```python
from build123d import *

# Parameters (mm, degrees)
SKETCH1_R           = 1.75
BOSS_EXTRUDE1_DEPTH = 6.25


with BuildPart() as part:
    # Sketch1 → Boss-Extrude1 (new, symmetric)
    with BuildSketch(Plane(origin=(0, 0, 0), x_dir=(1, 0, 0), z_dir=(0, 1, 0))):
        with Locations(Location((0, 0, 0), (0, 0, 270))):
            Circle(SKETCH1_R)
    extrude(amount=BOSS_EXTRUDE1_DEPTH, both=True)

    # Sketch2 → Revolve1 (revolve)
    with BuildSketch(Plane.XY, mode=Mode.PRIVATE) as revolve1_sk:
        with BuildLine():
            Line((-2.8, 6.25), (0, 6.25))
            Line((0, 6.25), (0, 7.75))
            Line((0, 7.75), (-2.8, 7.75))
            ThreePointArc((-2.8, 7.75), (-2.941421356, 7.691421356), (-3, 7.55))
            Line((-3, 7.55), (-3, 6.45))
            ThreePointArc((-3, 6.45), (-2.941421356, 6.308578644), (-2.8, 6.25))
        make_face()
        with BuildLine():
            Line((-2.8, -7.75), (0, -7.75))
            Line((0, -7.75), (0, -6.25))
            Line((0, -6.25), (-2.8, -6.25))
            ThreePointArc((-2.8, -6.25), (-2.941421356, -6.308578644), (-3, -6.45))
            Line((-3, -6.45), (-3, -7.55))
            ThreePointArc((-3, -7.55), (-2.941421356, -7.691421356), (-2.8, -7.75))
        make_face()
    revolve(revolve1_sk.sketch.rotate(Axis((0, -7.75, 0), (0, 1, 0)), 270), axis=Axis((0, -7.75, 0), (0, 1, 0)))


solid = part.part
```
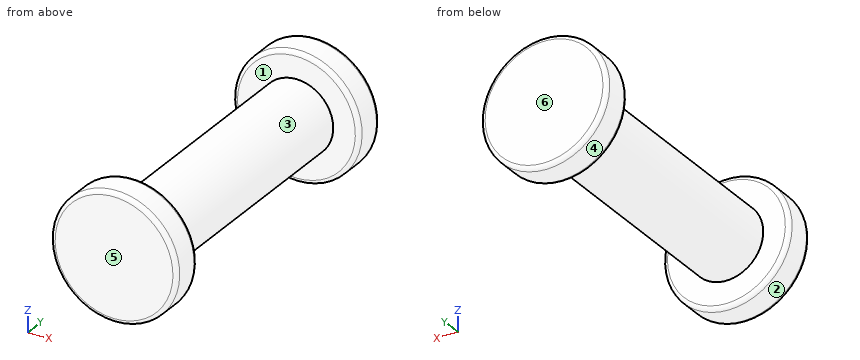
Here's how the part is built. I have some questions about the finished solid (model axes, mm). Face numbers are marked on the shaded views. A direction names the side the tool comes from. Round coordinates to 2 decimals unless told otherwise and drop trailing zeros. Loops run counter-clockwise (first coordinate to the right, second up) from the corner with the lowest first, then second, coordinate; pieces in that order, holes last.
1. Suppose I cut it at C-C, the plane y = -0.5. Please give me the cut outline in (x, z).
Answers:
outline: circle Ø3.5 at (0, 0)
2. Thinking about a two-plate mould opening in Y: for the marked faces 3, 4, 5 and 6, which applies, released by +Y, released by -Y, zero draft, split by the parting line, or undercut?
Answers:
face 3: undercut
face 4: zero draft
face 5: released by -Y
face 6: released by +Y
3. Suppose I cut it at A-A, the plane x = 0. Please give me the cut outline in (y, z).
Answers:
outline: (-7.75, -2.8) arc R0.2 ccw to (-7.55, -3) - (-6.45, -3) arc R0.2 ccw to (-6.25, -2.8) - (-6.25, -1.75) - (6.25, -1.75) - (6.25, -2.8) arc R0.2 ccw to (6.45, -3) - (7.55, -3) arc R0.2 ccw to (7.75, -2.8) - (7.75, 2.8) arc R0.2 ccw to (7.55, 3) - (6.45, 3) arc R0.2 ccw to (6.25, 2.8) - (6.25, 1.75) - (-6.25, 1.75) - (-6.25, 2.8) arc R0.2 ccw to (-6.45, 3) - (-7.55, 3) arc R0.2 ccw to (-7.75, 2.8) - close
4. For the marked faces 1 and 2, which set-ups out of +Z, -Z, +X, -X, +Y, -Y let a thin tool reach every point of the face, with its end or its side?
Answers:
face 1: none
face 2: +Y, -Y
5. If I drill on probe 1 along Y at (x, z) = (1.5, -1.5); probe 2 along X at (y, z) = (-5, 0.25); probe 3 along X at (y, z) = (-4.5, -1), over which ranges is the centre line in solid material (lowest first)?
Answers:
probe 1: y = -7.75 to -6.25, 6.25 to 7.75
probe 2: x = -1.73 to 1.73
probe 3: x = -1.44 to 1.44
6. Suppose I cut it at B-B, the plane z = 0. Please give me the cut outline in (x, y).
Answers:
outline: (-3, -7.55) arc R0.2 ccw to (-2.8, -7.75) - (2.8, -7.75) arc R0.2 ccw to (3, -7.55) - (3, -6.45) arc R0.2 ccw to (2.8, -6.25) - (1.75, -6.25) - (1.75, 6.25) - (2.8, 6.25) arc R0.2 ccw to (3, 6.45) - (3, 7.55) arc R0.2 ccw to (2.8, 7.75) - (-2.8, 7.75) arc R0.2 ccw to (-3, 7.55) - (-3, 6.45) arc R0.2 ccw to (-2.8, 6.25) - (-1.75, 6.25) - (-1.75, -6.25) - (-2.8, -6.25) arc R0.2 ccw to (-3, -6.45) - close
7. Will these pins go through, and if not, where does the flat tip stop? pin 1 (1.5 mm diameter, centred on x = -0.5, y = -4, fed in from +Z); pin 2 (3 mm diameter, centred on y = 1.5, z = -2, fed in from +X).
Answers:
pin 1: stops at z = 1.75
pin 2: stops at x = 1.68
